Could you check a few things on this model? Use its own coordinates, in mm. Face numbers are marked on the shaded views. A direction names the side the tool comes from. Round coordinates to 2 decimals unless told otherwise and drop trailing zeros. Loops run counter-clockwise (first coordinate to the right, second up) from the corner with the lowest first, then second, coordinate; pieces in that order, holes last. Notation, with made-up numbers: M 46.5,32.25 L 83.5,32.25 A5 cw 83.5,38.25 Z; hole C 31.25,-21 d6. An arc over 180 degrees is marked long. One line per item, written item: value. Start each with the question number.
Q1. Which directions (+Z, -Z, +X, -X, +Y, -Y) give clear straight access to the entire face, cutting with the end or side of a thin tool? Please do the marked faces 1, 2 and 3.
Q2. Please list where these lines run through material, in increasing order: line 1 along Z through (x, y) = (78, 761.5); line 2 along Z through (x, y) = (-76, 397.5).
Q3. I'm going to push flat-ended pins straight in: pin 1 Ø4 at (x, y) = (98.5, 312.5) entering from +Z; pin 2 Ø5 at (y, z) = (919, 162) entering from +X (3 decimals); pin 3 Ø5 at (x, y) = (9.5, 1095) entering from -Z. Where does each tip first touch, or does it pass through?
Q4. Imagine slicing it at D-D (y = 811.5). Please give me the cut outline in (x, z), then the cut area to 3 significant figures.
Q5. Imagine slicing it at C-C (z = 39.5). Please give me the cut outline in (x, y), then the cut area to 3 significant figures.
Q6. Thinking about a two-plate mould opening in Y: for the marked faces 4, 5 and 6, which applies, released by +Y, released by -Y, zero draft, split by the parting line, or undercut?
Q7. Imagine slicing it at B-B (x = -2). Give the number of separate pieces and of enclosed holes in the cut face, then the cut area to 3 significant figures.
Q8. Imagine slicing it at A-A (y = 463). Please give me the cut outline in (x, z).
from build123d import *

# Parameters (mm, degrees)
SKETCH1_W            = 600
SKETCH1_H            = 600
BOSS_EXTRUDE1_DEPTH  = 10
SKETCH2_W            = 600
SKETCH2_H            = 600
SKETCH2_W_2          = 560
SKETCH2_H_2          = 560
BOSS_AREA_C_DEPTH    = 590
SKETCH4_W            = 560
SKETCH4_H            = 20
CUT_AREA_C_DEPTH     = 590
SKETCH5_W            = 600
SKETCH5_H            = 600
SKETCH5_W_2          = 560
SKETCH5_H_2          = 560
AREA_B_DEPTH         = 300
SKETCH7_W            = 10
SKETCH7_H            = 590
CUT_EXTRUDE3_DEPTH   = 10
SKETCH8_W            = 220
SKETCH8_H            = 220
SKETCH8_W_2          = 200
SKETCH8_H_2          = 200
BOSS_EXTRUDE7_DEPTH  = 210
BOSS_EXTRUDE8_DEPTH  = 600
CUT_EXTRUDE4_DEPTH   = 600
BOSS_EXTRUDE9_DEPTH  = 600
CUT_EXTRUDE5_DEPTH   = 600
SKETCH16_W           = 231
SKETCH16_H           = 110
SKETCH16_W_2         = 210
SKETCH16_H_2         = 100
BOSS_EXTRUDE13_DEPTH = 25
SKETCH18_R           = 10
CUT_EXTRUDE6_DEPTH   = 35
FILLET1_R            = 5


with BuildPart() as part:
    # Sketch1 → Boss-Extrude1 (new body)
    with BuildSketch(Plane(origin=(0, 0, 0), x_dir=(1, 0, 0), z_dir=(0, 1, 0))):
        Rectangle(SKETCH1_W, SKETCH1_H)
    extrude(amount=BOSS_EXTRUDE1_DEPTH)

    # Sketch2 → Boss-Area C (add)
    with BuildSketch(Plane(origin=(0, 10, 0), x_dir=(1, 0, 0), z_dir=(0, 1, 0))):
        Rectangle(SKETCH2_W, SKETCH2_H)
        Rectangle(SKETCH2_W_2, SKETCH2_H_2, mode=Mode.SUBTRACT)
    extrude(amount=BOSS_AREA_C_DEPTH)

    # Sketch4 → Cut-Area C (cut)
    with BuildSketch(Plane(origin=(0, 600, 0), x_dir=(1, 0, 0), z_dir=(0, 1, 0))):
        with Locations((0, -290)):
            Rectangle(SKETCH4_W, SKETCH4_H)
    extrude(amount=-CUT_AREA_C_DEPTH, mode=Mode.SUBTRACT)

    # Sketch5 → Area B (add)
    with BuildSketch(Plane(origin=(0, 600, 0), x_dir=(1, 0, 0), z_dir=(0, 1, 0))):
        Rectangle(SKETCH5_W, SKETCH5_H)
        Rectangle(SKETCH5_W_2, SKETCH5_H_2, mode=Mode.SUBTRACT)
    extrude(amount=AREA_B_DEPTH)

    # Sketch7 → Cut-Extrude3 (cut)
    with BuildSketch(Plane.XY.offset(300)):
        with Locations((285, 305)):
            Rectangle(SKETCH7_W, SKETCH7_H)
        with Locations((-285, 305)):
            Rectangle(SKETCH7_W, SKETCH7_H)
    extrude(amount=-CUT_EXTRUDE3_DEPTH, mode=Mode.SUBTRACT)



with BuildPart() as body_2:
    # Sketch8 → Boss-Extrude7 (new body)
    with BuildSketch(Plane(origin=(0, 1100, 0), x_dir=(1, 0, 0), z_dir=(0, 1, 0))):
        Rectangle(SKETCH8_W, SKETCH8_H)
        Rectangle(SKETCH8_W_2, SKETCH8_H_2, mode=Mode.SUBTRACT)
    extrude(amount=-BOSS_EXTRUDE7_DEPTH)


with BuildPart() as part_1:
    add(part.part)

    add(body_2.part)  # Boss-Extrude8 merges body 2
    # Sketch9 → Boss-Extrude8 (add)
    with BuildSketch(Plane(origin=(0, 0, -300), x_dir=(-1, 0, 0), z_dir=(0, 0, -1))):
        Polygon((300, 900), (110, 1100), (110, 1090), (290, 900), align=None)
    boss_extrude8 = extrude(amount=-BOSS_EXTRUDE8_DEPTH)

    # Mirror1: Boss-Extrude8 across plane
    add(boss_extrude8.mirror(Plane(origin=(0, 0, 0), x_dir=(0, 0, 1), z_dir=(1, 0, 0))))

    # Sketch10 → Cut-Extrude4 (cut)
    with BuildSketch(Plane.ZY.offset(300)):
        Polygon((-300, 900), (-300, 1100), (-110, 1100), align=None)
        Polygon((300, 1100), (110, 1100), (300, 900), align=None)
    extrude(amount=-CUT_EXTRUDE4_DEPTH, mode=Mode.SUBTRACT)

    # Sketch13 → Boss-Extrude9 (add)
    with BuildSketch(Plane(origin=(300, 0, 0), x_dir=(0, 0, -1), z_dir=(1, 0, 0))):
        Polygon((-300, 900), (-290, 900), (-110.315522005, 1090), (-110.315522005, 1100), align=None)
        Polygon((300, 900), (290, 900), (110.315522005, 1090), (110.315522005, 1100), align=None)
    extrude(amount=-BOSS_EXTRUDE9_DEPTH)

    # Sketch14 → Cut-Extrude5 (cut)
    with BuildSketch(Plane(origin=(0, 0, -300), x_dir=(-1, 0, 0), z_dir=(0, 0, -1))):
        Polygon((-110, 1100), (-300, 900), (-300, 1100), align=None)
        Polygon((300, 1100), (110, 1100), (300, 900), align=None)
    extrude(amount=-CUT_EXTRUDE5_DEPTH, mode=Mode.SUBTRACT)

    # Sketch16 → Boss-Extrude13 (add)
    with BuildSketch(Plane(origin=(0, 575.982283096, -607.305657461), x_dir=(-1, 0, 0), z_dir=(0, 0.6881475597150754, -0.7255707657135773))):
        with Locations((0, 584.806743705)):
            Rectangle(SKETCH16_W, SKETCH16_H)
        with Locations((0, 584.806743705)):
            Rectangle(SKETCH16_W_2, SKETCH16_H_2, mode=Mode.SUBTRACT)
    extrude(amount=BOSS_EXTRUDE13_DEPTH)

    # Sketch18 → Cut-Extrude6 (cut)
    with BuildSketch(Plane(origin=(0, 575.982283096, -607.305657461), x_dir=(-1, 0, 0), z_dir=(0, 0.6881475597150754, -0.7255707657135773))):
        with Locations(Location((-35, 584.806743705, 0), (0, 0, 90))):
            Circle(SKETCH18_R)
        with Locations(Location((35, 584.806743705, 0), (0, 0, 90))):
            Circle(SKETCH18_R)
    extrude(amount=-CUT_EXTRUDE6_DEPTH, mode=Mode.SUBTRACT)

    # Fillet1
    fillet1_edges = [part_1.edges().sort_by_distance(p)[0] for p in [
        (300, 450, 300),
        (-300, 450, 300),
        (-300, 450, -300),
        (300, 450, -300),
    ]]
    fillet(fillet1_edges, radius=FILLET1_R)


solid = part_1.part
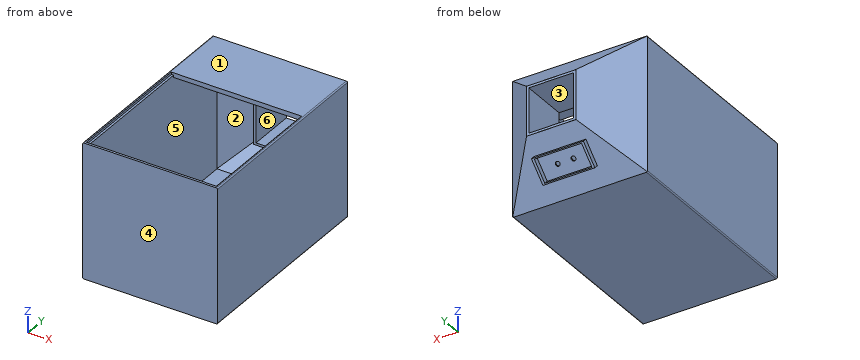
Report:
1. face 1: +Z, +X, -X, +Y, -Y
1. face 2: none
1. face 3: +Y
2. line 1: z = -300 to -280, 280 to 300
2. line 2: z = -300 to -280
3. pin 1: stops at z = -280
3. pin 2: stops at x = 284.325
3. pin 3: stops at z = -117.43
4. outline: M -300,-295 A5 ccw -295,-300 L 295,-300 A5 ccw 300,-295 L 300,295 A5 ccw 295,300 L -295,300 A5 ccw -300,295 Z; hole M -280,-280 L 280,-280 L 280,280 L -280,280 Z
4. area: 46,400 mm²
5. outline: M -300,0 L 300,0 L 300,900 L 110,1100 L 100,1100 L 100,890 L 110,890 L 110,1090 L 290,900 L 280,900 L 280,10 L -280,10 L -280,900 L -290,900 L -110,1090 L -110,890 L -100,890 L -100,1100 L -110,1100 L -300,900 Z
5. area: 49,600 mm²
6. face 4: released by -Y
6. face 5: undercut
6. face 6: zero draft
7. separate pieces: 4
7. enclosed holes: 0
7. area: 38,000 mm²
8. outline: M -300,-295 A5 ccw -295,-300 L 295,-300 A5 ccw 300,-295 L 300,295 A5 ccw 295,300 L 290,300 L 290,290 L 280,290 L 280,-280 L -280,-280 L -280,290 L -290,290 L -290,300 L -295,300 A5 ccw -300,295 Z
